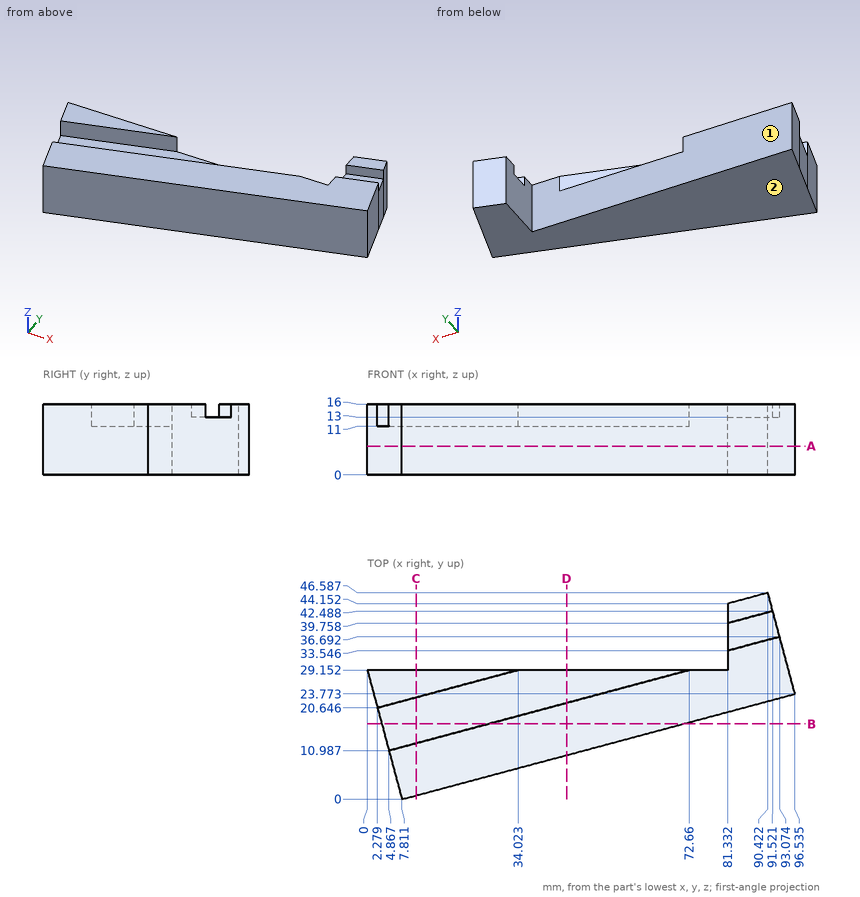
Check sheet for the drawn part. Datum: minimum x, y, z corner. Units: mm. A direction names the side the tool comes from. Coordinates: 2 decimals unless noted, no trailing zeros. Loops run counter-clockwise (first coordinate to the right, second up) from the corner with the lowest first, then second, coordinate; pieces in that order, holes last. Notation, with made-up numbers: (-20.75, -12.5) -> (33.25, -12.5) arc R14 cw to (33.25, -8.5) -> close; hole circle Ø3 at (78, -10.5). An arc over 180 degrees is marked (long way). Answer in a Markdown table with one row per item.
1. Sectioned sample at C-C, the plane x = 11. Record the boundary of the cut face in (y, z) (1 decimal), then the cut area to 3 significant figures.
Check values:
| item | result |
|---|---|
| outline | (0.9, 0) -> (29.2, 0) -> (29.2, 16) -> (23, 16) -> (23, 11) -> (12.6, 11) -> (12.6, 16) -> (0.9, 16) -> close |
| area | 401 mm2 |
2. Material ranges on line 1 along Y through (x, z) = (24, 12.25) (1 decimal); line 2 along Y through (x, z) = (54.5, 2.75); line 3 along Y through (x, z) = (9, 11.25) (1 decimal), recorded low to high. Write a range as [from, to].
Check values:
| item | result |
|---|---|
| line 1 | y = [4.3, 16.1], [26.5, 29.2] |
| line 2 | y = [12.51, 29.15] |
| line 3 | y = [0.3, 12.1], [22.4, 29.2] |
3. Sectioned sample at A-A, the plane z = 6.5. Record the boundary of the cut face in (x, y) (1 decimal).
Check values:
| item | result |
|---|---|
| outline | (0, 29.2) -> (7.8, 0) -> (96.5, 23.8) -> (90.4, 46.6) -> (81.3, 44.2) -> (81.3, 29.2) -> close |
4. Go/stop test with flat-tipped pins: pin 1 (3 mm diameter, centred on x = 31.5, z = 5.5, fed in from -Y) (1 decimal); pin 2 (7.5 mm diameter, centred on y = 39, z = 10.5, fed in from -X); pin 3 (5 mm diameter, centred on x = 20.5, z = 7.5, fed in from +Y). Record where each tip stops, or that it passes through.
Check values:
| item | result |
|---|---|
| pin 1 | stops at y = 5.9 |
| pin 2 | stops at x = 81.33 |
| pin 3 | stops at y = 29.15 |
5. Sectioned sample at B-B, the plane y = 17. Record the boundary of the cut face in (x, z).
Check values:
| item | result |
|---|---|
| outline | (3.26, 0) -> (71.26, 0) -> (71.26, 16) -> (27.31, 16) -> (27.31, 11) -> (3.26, 11) -> close |
6. Access from +Z, -Z, +X, -X, +Y, -Y to the whole of each face (thin tool, end or side, straight path). Record for the marked faces 1 and 2.
Check values:
| item | result |
|---|---|
| face 1 | +Z, -Z, -X, +Y |
| face 2 | -Z, +X, -X, +Y, -Y |
7. Sectioned sample at D-D, the plane x = 45. Record the boundary of the cut face in (y, z) (1 decimal).
Check values:
| item | result |
|---|---|
| outline | (10, 0) -> (29.2, 0) -> (29.2, 11) -> (21.7, 11) -> (21.7, 16) -> (10, 16) -> close |
